Work out the finished part from the listing and answer in its coordinate system (mm). Face numbers are marked on the shaded views. A direction names the side the tool comes from. Give positions to 0.01 mm unless a question says otherwise; leave off trailing zeros. Loops run counter-clockwise (first coordinate to the right, second up) from the corner with the lowest first, then second, coordinate; pieces in that order, holes last. Notation, with made-up numbers: (-13, -29) - (17, -29) arc R29 cw to (17, 6) - close; hole circle Ø6 at (7.5, 76). An arc over 180 degrees is marked (long way). Use CSV: the item, a comma, the result in double quotes.
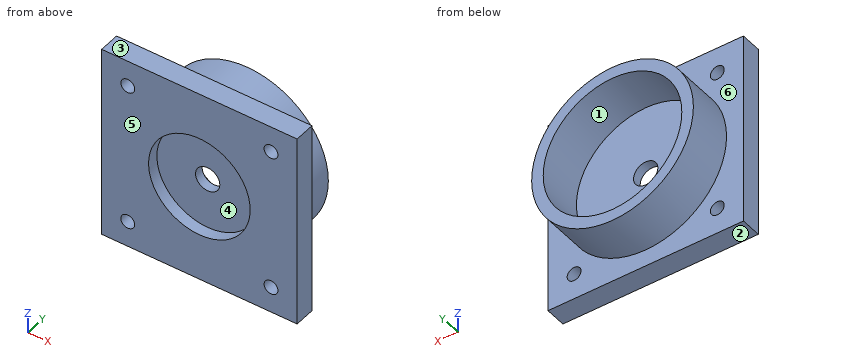
from build123d import *

# Parameters (mm, degrees)
SKETCH1_W           = 42.3
SKETCH1_H           = 42.3
SKETCH1_R           = 1.5
BOSS_EXTRUDE1_DEPTH = 4.5
SKETCH2_R           = 11
CUT_EXTRUDE1_DEPTH  = 2.5
SKETCH3_R           = 2.625
CUT_EXTRUDE2_DEPTH  = 2
SKETCH4_R           = 17.5
SKETCH4_R_2         = 15
BOSS_EXTRUDE2_DEPTH = 10


with BuildPart() as part:
    # Sketch1 → Boss-Extrude1 (new body)
    with BuildSketch(Plane(origin=(0, 0, 0), x_dir=(1, 0, 0), z_dir=(0, 1, 0))):
        Rectangle(SKETCH1_W, SKETCH1_H)
        with Locations(Location((-15.5, 15.5, 0), (0, 0, 270))):
            Circle(SKETCH1_R, mode=Mode.SUBTRACT)
        with Locations(Location((15.5, 15.5, 0), (0, 0, 270))):
            Circle(SKETCH1_R, mode=Mode.SUBTRACT)
        with Locations(Location((-15.5, -15.5, 0), (0, 0, 270))):
            Circle(SKETCH1_R, mode=Mode.SUBTRACT)
        with Locations(Location((15.5, -15.5, 0), (0, 0, 270))):
            Circle(SKETCH1_R, mode=Mode.SUBTRACT)
    extrude(amount=BOSS_EXTRUDE1_DEPTH)

    # Sketch2 → Cut-Extrude1 (cut)
    with BuildSketch(Plane.XZ):
        with Locations(Location((0, 0, 0), (0, 0, 270))):
            Circle(SKETCH2_R)
    extrude(amount=-CUT_EXTRUDE1_DEPTH, mode=Mode.SUBTRACT)

    # Sketch3 → Cut-Extrude2 (cut)
    with BuildSketch(Plane.XZ.offset(-2.5)):
        with Locations(Location((0, 0, 0), (0, 0, 270))):
            Circle(SKETCH3_R)
    extrude(amount=-CUT_EXTRUDE2_DEPTH, mode=Mode.SUBTRACT)

    # Sketch4 → Boss-Extrude2 (add)
    with BuildSketch(Plane(origin=(0, 4.5, 0), x_dir=(1, 0, 0), z_dir=(0, 1, 0))):
        with Locations(Location((0, 0, 0), (0, 0, 90))):
            Circle(SKETCH4_R)
        with Locations(Location((0, 0, 0), (0, 0, 270))):
            Circle(SKETCH4_R_2, mode=Mode.SUBTRACT)
    extrude(amount=BOSS_EXTRUDE2_DEPTH)


solid = part.part
Item 1: For the marked faces 5 and 6, determine the directions among +Z, -Z, +X, -X, +Y, -Y from which every point of the face is accessible in a straight line to the end or side of a thin tool.
Determined:
face 5,"+Z, -Z, +X, -X, -Y"
face 6,"+Y"
Item 2: Find the intervals of material crossed by line 1 (X direction, y = 2.5, z = -15.5); line 2 (X direction, y = 0.5, z = 0); line 3 (X direction, y = 1.75, z = -16), in increasing order.
Determined:
line 1,"x = -21.15 to -17, -14 to 14, 17 to 21.15"
line 2,"x = -21.15 to -11, 11 to 21.15"
line 3,"x = -21.15 to -16.91, -14.09 to 14.09, 16.91 to 21.15"
Item 3: The mould has two halves that part along Z. Classify the marked faces 1, 2, 3 and 4: pulls with the +Z half, pulls with the -Z half, needs draft (parallel to the pull), parting line crosses it, or undercut.
Determined:
face 1,"undercut"
face 2,"pulls with the -Z half"
face 3,"pulls with the +Z half"
face 4,"undercut"
Item 4: A cutting plane is placed at D-D on z = 0.5. Determine the outline of the cut face in (x, y), and give its area (3 significant figures).
Determined:
outline,"(-21.15, 0) - (-10.99, 0) - (-10.99, 2.5) - (-2.58, 2.5) - (-2.58, 4.5) - (-14.99, 4.5) - (-14.99, 14.5) - (-17.49, 14.5) - (-17.49, 4.5) - (-21.15, 4.5) - close; (2.58, 2.5) - (10.99, 2.5) - (10.99, 0) - (21.15, 0) - (21.15, 4.5) - (17.49, 4.5) - (17.49, 14.5) - (14.99, 14.5) - (14.99, 4.5) - (2.58, 4.5) - close"
area,"175 mm²"
Item 5: A cutting plane is placed at A-A on x = 0. Determine the outline of the cut face in (y, z) (3 decimals).
Determined:
outline,"(0, -21.15) - (4.5, -21.15) - (4.5, -17.5) - (14.5, -17.5) - (14.5, -15) - (4.5, -15) - (4.5, -2.625) - (2.5, -2.625) - (2.5, -11) - (0, -11) - close; (0, 11) - (2.5, 11) - (2.5, 2.625) - (4.5, 2.625) - (4.5, 15) - (14.5, 15) - (14.5, 17.5) - (4.5, 17.5) - (4.5, 21.15) - (0, 21.15) - close"
Item 6: Given P1, Ø17.5, axis at x = -1.5, z = -1, coming from the -Y side; P2, Ø4, axis at x = 3.5, y = 7.5, coming from the +Z side; P3, Ø4, axis at x = -4, y = 10, coming from the -Z side; P4, Ø24, axis at x = -6.5, z = 3.5, coming from the +Y side, each flat-ended and moving along its own axis, determine where each tip first touches the part or whether it passes through.
Determined:
P1,"stops at y = 2.5"
P2,"stops at z = 17.44"
P3,"stops at z = -17.39"
P4,"stops at y = 14.5"
Item 7: A cutting plane is placed at C-C on z = 16. Determine the outline of the cut face in (x, y), and give its area (3 significant figures).
Determined:
outline,"(-21.15, 0) - (-16.91, 0) - (-16.91, 4.5) - (-21.15, 4.5) - close; (-14.09, 0) - (14.09, 0) - (14.09, 4.5) - (7.09, 4.5) - (7.09, 14.5) - (-7.09, 14.5) - (-7.09, 4.5) - (-14.09, 4.5) - close; (16.91, 0) - (21.15, 0) - (21.15, 4.5) - (16.91, 4.5) - close"
area,"307 mm²"
Item 8: A cutting plane is placed at B-B on x = 15.5. Determine the outline of the cut face in (y, z).
Determined:
outline,"(0, -21.15) - (4.5, -21.15) - (4.5, -17) - (0, -17) - close; (0, -14) - (4.5, -14) - (4.5, -8.12) - (14.5, -8.12) - (14.5, 8.12) - (4.5, 8.12) - (4.5, 14) - (0, 14) - close; (0, 17) - (4.5, 17) - (4.5, 21.15) - (0, 21.15) - close"
